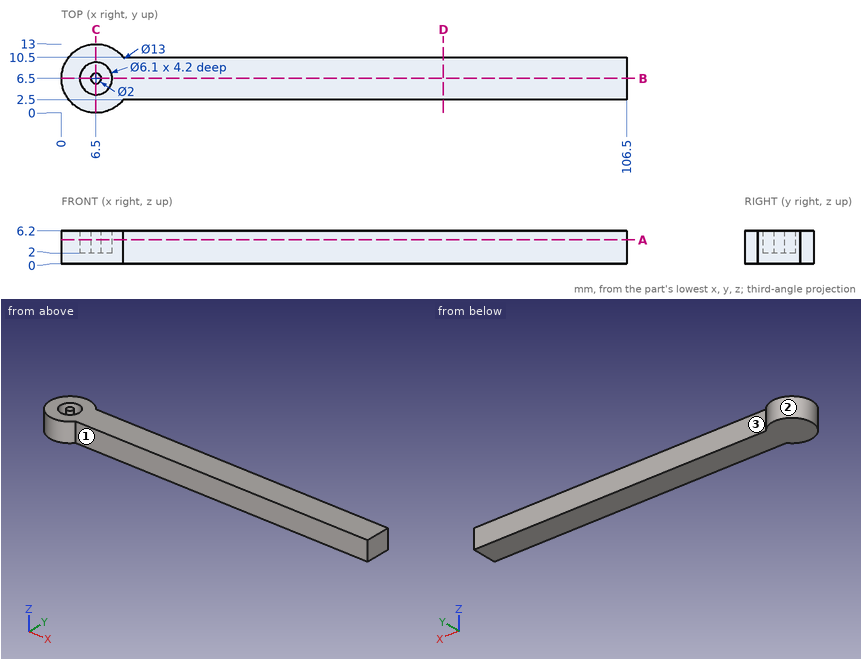
The figure shows three views and two pictorial views of one solid part (mm, origin at its lowest corner). Answer the questions. A direction names the side the tool comes from. Coordinates: 2 decimals unless noted, no trailing zeros. Loops run counter-clockwise (first coordinate to the right, second up) from the corner with the lowest first, then second, coordinate; pieces in that order, holes last. Notation, with made-up numbers: (-5.5, 21.25) - (52.5, 21.25) arc R23 cw to (52.5, 37.25) - close; hole circle Ø2 at (54.25, -1). An arc over 180 degrees is marked (long way). Use a Markdown table: item, result. Add a question column.
1) For the marked faces 1, 2 and 3, determine the directions among +Z, -Z, +X, -X, +Y, -Y from which every point of the face is accessible in a straight line to the end or side of a thin tool.
2) The part is cut by section D-D, the plane x = 72. Give the vertices of the cut face in (y, z), and give its area (3 significant figures).
3) The part is cut by section B-B, the plane y = 6.5. Give the vertices of the cut face in (x, z), and give its area (3 significant figures).
4) Given pin 1 (1 mm diameter, centred on x = 65.5, z = 2, fed in from -Y); pin 2 (3 mm diameter, centred on x = 18.5, z = 4.5, fed in from +Y), each flat-ended and moving along its own axis, determine where each tip first touches the part or whether it passes through.
5) The part is cut by section A-A, the plane z = 4.5. Give the vertices of the cut face in (x, y).
6) Find the intervals of material crossed by line 1 (Y direction, x = 6.5, z = 3.15); line 2 (Y direction, x = 19.5, z = 0.5); line 3 (X direction, y = 4.5, z = 3), in increasing order.
7) The part is cut by section C-C, the plane x = 6.5. Give the vertices of the cut face in (y, z).
Here are the results:
| question | item | result |
|---|---|---|
| 1 | face 1 | +Z, -Z, +X, -Y |
| 1 | face 2 | +Z, -Z |
| 1 | face 3 | +Z, -Z, +X, +Y |
| 2 | outline | (2.5, 0) - (10.5, 0) - (10.5, 6.2) - (2.5, 6.2) - close |
| 2 | area | 49.6 mm^2 |
| 3 | outline | (0, 0) - (106.5, 0) - (106.5, 6.2) - (9.55, 6.2) - (9.55, 2) - (7.5, 2) - (7.5, 6.2) - (5.5, 6.2) - (5.5, 2) - (3.45, 2) - (3.45, 6.2) - (0, 6.2) - close |
| 3 | area | 643 mm^2 |
| 4 | pin 1 | stops at y = 2.5 |
| 4 | pin 2 | stops at y = 10.5 |
| 5 | outline | circle Ø2 at (6.5, 6.5); (11.62, 2.5) - (106.5, 2.5) - (106.5, 10.5) - (11.62, 10.5) arc R6.5 ccw (long way) to start; hole circle Ø6.1 at (6.5, 6.5) |
| 6 | line 1 | y = 0 to 3.45, 5.5 to 7.5, 9.55 to 13 |
| 6 | line 2 | y = 2.5 to 10.5 |
| 6 | line 3 | x = 0.32 to 4.2, 8.8 to 106.5 |
| 7 | outline | (0, 0) - (13, 0) - (13, 6.2) - (9.55, 6.2) - (9.55, 2) - (7.5, 2) - (7.5, 6.2) - (5.5, 6.2) - (5.5, 2) - (3.45, 2) - (3.45, 6.2) - (0, 6.2) - close |
